Could you check a few things on this drawing? It's one solid part, dimensions in mm from its lowest x, y, z. A direction names the side the tool comes from. Give positions to 0.01 mm unless a question says otherwise; leave off trailing zeros. Loops run counter-clockwise (first coordinate to the right, second up) from the corner with the lowest first, then second, coordinate; pieces in that order, holes last. Notation, with made-up numbers: M 87,16.5 L 140,16.5 A21 cw 140,41.5 Z; hole C 3.25,80.25 d1. An arc over 180 degrees is marked long. Return JSON: item names as keys, results as strings. Group by question number.
1. Please list where these lines run through material, in increasing order: line 1 (X direction, y = 2.25, z = 9.5); line 2 (X direction, y = 35.5, z = 14.5); line 3 (Y direction, x = 35.5, z = 9.5).
2. If we mould it in two halves opening along Y, with no side actions, what happens to the marked faces 1, 2, 3 and 4? For each: +Y half, -Y half, draft (parallel to the pull), parting line (faces both ways), or undercut.
3. For the marked faces 5, 6 and 7, which set-ups out of +Z, -Z, +X, -X, +Y, -Y let a thin tool reach every point of the face, with its end or its side?
4. If we section it at C-C (y = 25): Write out the boundary of the cut face in (x, z).
5. If we section it at A-A (x = 13): Write out the boundary of the cut face in (y, z).
6. For pin 1 (4.5 mm diameter, centred on y = 26, z = 16, fed in from -X); pin 2 (1.7 mm diameter, centred on y = 24, z = 2.5, fed in from +X); pin 3 (1 mm diameter, centred on y = 6.5, z = 15, fed in from -X); pin 4 (6 mm diameter, centred on x = 13, z = 9.5, fed in from -Y), each with a flat end and sliding along its axis, tell me the tip position at first contact or that it passes through.
7. If we section it at B-B (z = 9.5): Write out the boundary of the cut face in (x, y).
8. If we section it at D-D (x = 33.5): Write out the boundary of the cut face in (y, z).
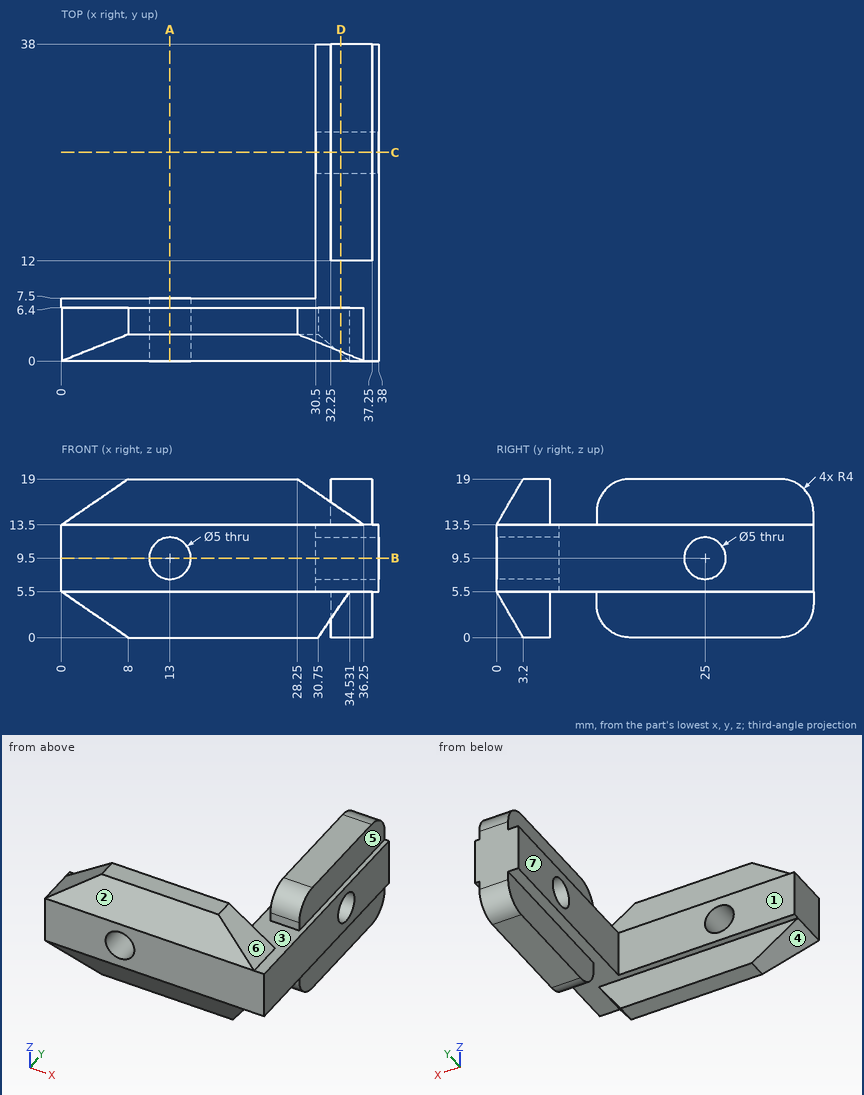
Answer:
{
 "1": {"line 1": "x = 0 to 10.5, 15.5 to 38", "line 2": "x = 32.25 to 37.25", "line 3": "y = 0 to 22.5, 27.5 to 38"},
 "2": {"face 1": "+Y half", "face 2": "-Y half", "face 3": "undercut", "face 4": "draft"},
 "3": {"face 5": "+Z, +X, +Y, -Y", "face 6": "+Z, +X, -Y", "face 7": "+Z, -Z, -X, +Y"},
 "4": {"outline": "M 30.5,5.5 L 32.25,5.5 L 32.25,0 L 37.25,0 L 37.25,5.5 L 38,5.5 L 38,7 L 30.5,7 Z; M 30.5,12 L 38,12 L 38,13.5 L 37.25,13.5 L 37.25,19 L 32.25,19 L 32.25,13.5 L 30.5,13.5 Z"},
 "5": {"outline": "M 0,5.5 L 3.2,0 L 6.4,0 L 6.4,5.5 L 7.5,5.5 L 7.5,7 L 0,7 Z; M 0,12 L 7.5,12 L 7.5,13.5 L 6.4,13.5 L 6.4,19 L 3.2,19 L 0,13.5 Z"},
 "6": {"pin 1": "stops at x = 32.25", "pin 2": "stops at x = 37.25", "pin 3": "stops at x = 1.47", "pin 4": "stops at y = 0"},
 "7": {"outline": "M 0,0 L 10.5,0 L 10.5,7.5 L 0,7.5 Z; M 15.5,0 L 38,0 L 38,22.5 L 30.5,22.5 L 30.5,7.5 L 15.5,7.5 Z; M 30.5,27.5 L 38,27.5 L 38,38 L 30.5,38 Z"},
 "8": {"outline": "M 0,5.5 L 0.87,4 L 6.4,4 L 6.4,5.5 L 12,5.5 L 12,4 A4 ccw 16,0 L 34,0 A4 ccw 38,4 L 38,15 A4 ccw 34,19 L 16,19 A4 ccw 12,15 L 12,13.5 L 6.4,13.5 L 6.4,15.39 L 1.1,15.39 L 0,13.5 Z; hole C 25,9.5 d5"}
}
